from build123d import *

# Parameters (mm, degrees)
F1_DEPTH = 50.8
F2_T     = -6.35
F3_W     = 91.786147
F3_H     = 76.2
F4_DEPTH = 6.35


with BuildPart() as f1:
    # F0 (on Front) → F1 (new body)
    with BuildSketch(Plane.XZ):
        Polygon((38.380861, 43.561175), (-19.363867, 43.561175), (-40.705286, 21.657981), (-40.705286, -38.248271), (38.380861, -38.248271), align=None)
    extrude(amount=F1_DEPTH)

    # F2
    f2_openings = [f1.faces().sort_by_distance(p)[0] for p in [
        (38.380861, -25.4, 2.656452),
        (-1.162212, -25.4, -38.248271),
    ]]
    offset(amount=F2_T, openings=f2_openings)

    # F3 (on face) → F4 (join)
    with BuildSketch(Plane(origin=(0, 0, -38.248271), x_dir=(1, 0, 0), z_dir=(0, 0, -1))):
        with Locations((-7.512213, 25.4)):
            Rectangle(F3_W, F3_H)
    extrude(amount=F4_DEPTH)


solid = f1.part
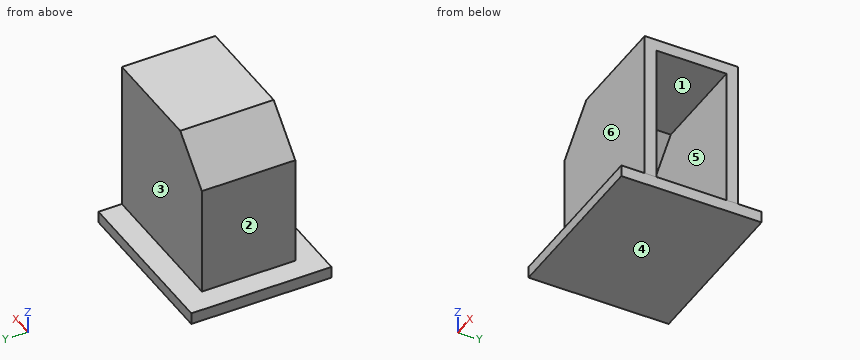
Could you check a few things on this model? Use its own coordinates, in mm. Face numbers are marked on the shaded views. A direction names the side the tool comes from. Coordinates: 2 decimals unless noted, no trailing zeros. Loops run counter-clockwise (first coordinate to the right, second up) from the corner with the lowest first, then second, coordinate; pieces in that order, holes last.
1. We'd pull the mould along Z, two halves only. Please class the marked faces 4, 5 and 6: released by +Z, released by -Z, zero draft, split by the parting line, or undercut.
2. Imagine slicing it at A-A (x = 25.5). Please give me the cut outline in (y, z), and give its area (3 significant figures).
3. Imagine slicing it at C-C (y = -26.5). Please give me the cut outline in (x, z).
4. Imagine slicing it at D-D (x = -45.5). Please give me the cut outline in (y, z), and give its area (3 significant figures).
5. For P1, Ø8, axis at x = -36, z = -4, coming from the -Y side; P2, Ø1, axis at x = -38, y = -15, coming from the +Z side; P3, Ø4, axis at y = -42, z = 14.5, coming from the +X side; P4, Ø1, axis at y = 1, z = 17.5, coming from the +X side, each with a flat end and sliding along its axis, tell me the tip position at first contact or that it passes through.
6. I need wall thicknesses on L1, parallel to Y at x = 34.5, z = 23; L2, parallel to Z at x = -2, y = -26; L3, parallel to Y at x = -36.5, z = 0. Which ranges of each line are inside material? Lowest first, please.
7. For the marked faces 1, 2 and 3, which set-ups out of +Z, -Z, +X, -X, +Y, -Y let a thin tool reach every point of the face, with its end or its side?
8. Imagine slicing it at B-B (z = -35). Please give me the cut outline in (x, y).
Computed values:
1. face 4: released by -Z
1. face 5: undercut
1. face 6: zero draft
2. outline: (-63.5, -44.6) - (12.7, -44.6) - (12.7, -38.25) - (0, -38.25) - (0, 43.56) - (-50.8, 43.56) - (-50.8, -38.25) - (-63.5, -38.25) - close; hole (-44.45, -38.25) - (-6.35, -38.25) - (-6.35, 37.21) - (-44.45, 37.21) - close
2. area: 1,760 mm2
3. outline: (-53.41, -44.6) - (38.38, -44.6) - (38.38, -38.25) - (-34.36, -38.25) - (-34.36, 19.08) - (-16.69, 37.21) - (38.38, 37.21) - (38.38, 43.56) - (-19.36, 43.56) - (-40.71, 21.66) - (-40.71, -38.25) - (-53.41, -38.25) - close
4. outline: (-63.5, -44.6) - (12.7, -44.6) - (12.7, -38.25) - (-63.5, -38.25) - close
4. area: 484 mm2
5. P1: stops at y = -50.8
5. P2: stops at z = 24.95
5. P3: stops at x = -34.36
5. P4: passes through
6. L1: y = -50.8 to -44.45, -6.35 to 0
6. L2: z = -44.6 to -38.25, 37.21 to 43.56
6. L3: y = -50.8 to 0
7. face 1: +X
7. face 2: +Z, -X, +Y, -Y
7. face 3: +Z, +X, -X, +Y
8. outline: (-40.71, -50.8) - (38.38, -50.8) - (38.38, -44.45) - (-34.36, -44.45) - (-34.36, -6.35) - (38.38, -6.35) - (38.38, 0) - (-40.71, 0) - close
